Source: three-view drawing plus pictorial views. Frame: mm from the lowest corner of the part. Coordinates: 2 decimals unless noted, no trailing zeros. Order: outer loops, then holes, each group sorted by start corner. A loop starts at its lowest first (then second) coordinate and runs counter-clockwise, first axis right, second up. Notation, with made-up numbers: (38, 47.5) - (77, 47.5) arc R25 cw to (77, 69.5) - close; hole circle Ø1 at (57.5, 7.25). An arc over 180 degrees is marked (long way). One line per question, with ' | ' between items.
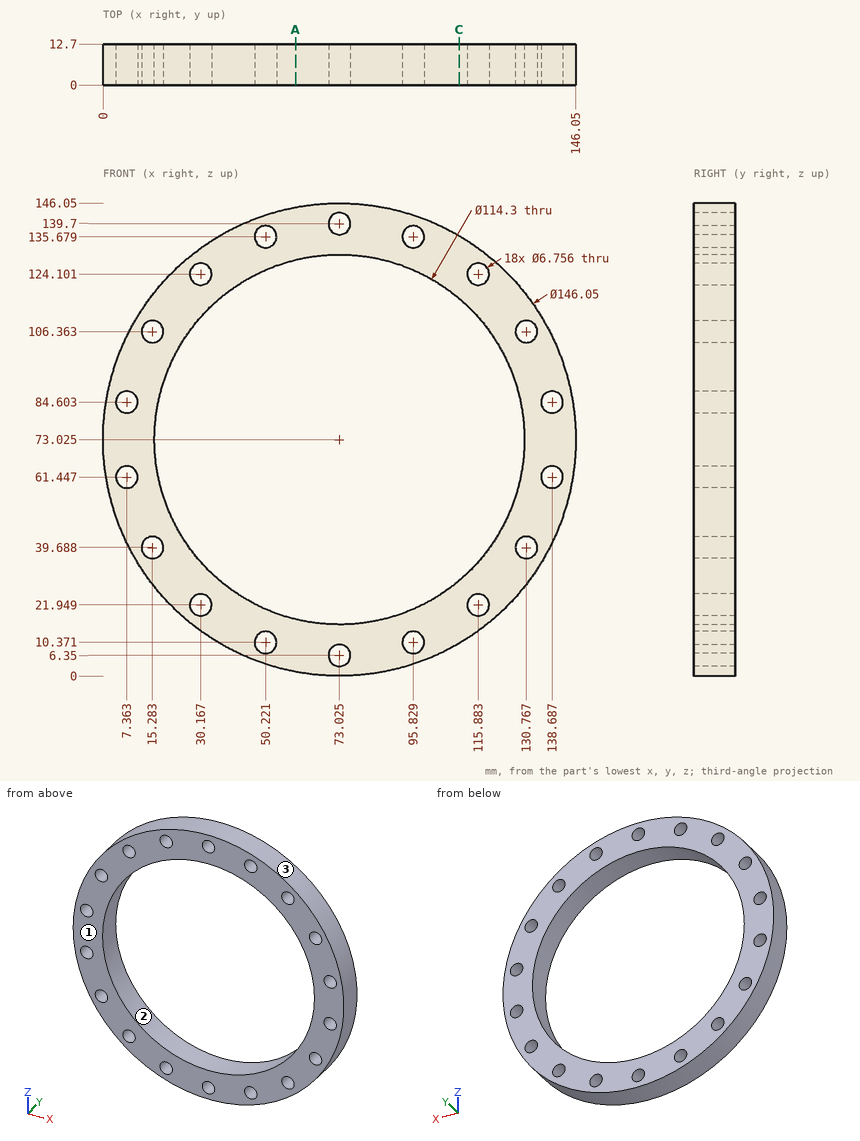
(1) Cut plane C-C (x = 110). Return the cut outline in (y, z).
Taken from the geometry:
outline: (0, 10.05) - (12.7, 10.05) - (12.7, 29.45) - (0, 29.45) - close; (0, 116.6) - (12.7, 116.6) - (12.7, 136) - (0, 136) - close
(2) Pin query (flat end, axial travel): P1, Ø1, axis at y = 10, z = 95, coming from the +X side; P2, Ø9, axis at x = 30.17, z = 21.95, coming from the -Y side; P3, Ø1.5, axis at x = 83, y = 5.5, coming from the +Z side (1 decimal); P4, Ø6, axis at x = 94, y = 3.5, coming from the -Z side. Return the tip coordinate at first contact, or that it passes through.
Taken from the geometry:
P1: stops at x = 142.82 | P2: stops at y = 0 | P3: stops at z = 145.5 | P4: stops at z = 2.25
(3) Cut plane A-A (x = 59.5). Return the cut outline in (y, z), and give its area (3 significant figures).
Taken from the geometry:
outline: (0, 1.26) - (12.7, 1.26) - (12.7, 17.5) - (0, 17.5) - close; (0, 128.55) - (12.7, 128.55) - (12.7, 144.79) - (0, 144.79) - close | area: 412 mm²
(4) Material intervals for L1, parallel to X at y = 9.5, z = 72.5; L2, parallel to Z at x = 14, y = 5.25 (1 decimal); L3, parallel to Z at x = 48, y = 3.75 (1 decimal), sorted ascending. Write a range as from..to.
Taken from the geometry:
L1: x = 0..15.88, 130.17..146.05 | L2: z = 30..36.6, 42.8..103.2, 109.5..116 | L3: z = 4.4..7.8, 12.9..21.6, 124.4..133.1, 138.2..141.6
(5) Pull-direction query (Z, two-part tool) for the marked faces 1, 2 and 3; classes: pulls with the +Z half, pulls with the -Z half, needs draft (parallel to the pull), parting line crosses it, or undercut.
Taken from the geometry:
face 1: needs draft | face 2: undercut | face 3: parting line crosses it
